```python
from build123d import *

# Parameters (mm, degrees)
SKETCH1_W           = 19.05
SKETCH1_H           = 38.1
SKETCH1_R           = 1.905
BOSS_EXTRUDE1_DEPTH = 3.81
BOSS_EXTRUDE2_DEPTH = 6.35
SKETCH3_W           = 10.16
SKETCH3_H           = 38.1
BOSS_EXTRUDE3_DEPTH = 2.54
CHAMFER1_SIZE       = 1.27


with BuildPart() as part:
    # Sketch1 → Boss-Extrude1 (new body)
    with BuildSketch(Plane(origin=(0, 0, 0), x_dir=(1, 0, 0), z_dir=(0, 1, 0))):
        with Locations((-4.445, -12.7)):
            Rectangle(SKETCH1_W, SKETCH1_H)
        with Locations(Location((0, 0, 0), (0, 0, 90))):
            Circle(SKETCH1_R, mode=Mode.SUBTRACT)
        with Locations(Location((0, -25.4, 0), (0, 0, 90))):
            Circle(SKETCH1_R, mode=Mode.SUBTRACT)
    extrude(amount=BOSS_EXTRUDE1_DEPTH)

    # Sketch2 → Boss-Extrude2 (add)
    with BuildSketch(Plane(origin=(0, 3.81, 0), x_dir=(1, 0, 0), z_dir=(0, 1, 0))):
        Polygon((-13.97, 6.35), (-13.97, -31.75), (-3.81, -31.75), (-3.81, 6.35), (-6.35, 6.35), (-6.35, -29.21), (-11.43, -29.21), (-11.43, 6.35), align=None)
    extrude(amount=BOSS_EXTRUDE2_DEPTH)

    # Sketch3 → Boss-Extrude3 (add)
    with BuildSketch(Plane(origin=(0, 10.16, 0), x_dir=(1, 0, 0), z_dir=(0, 1, 0))):
        with Locations((-8.89, -12.7)):
            Rectangle(SKETCH3_W, SKETCH3_H)
    extrude(amount=BOSS_EXTRUDE3_DEPTH)

    # Chamfer1
    chamfer1_edges = [part.edges().sort_by_distance(p)[0] for p in [
        (-6.35, 10.16, 11.43),
        (-11.43, 10.16, 11.43),
    ]]
    chamfer(chamfer1_edges, length=CHAMFER1_SIZE)


with BuildPart() as body_2:
    # Mirror1: mirrored copy
    add(part.part.mirror(Plane(origin=(5.08, 3.81, -6.35), x_dir=(0, 0, 1), z_dir=(-1, 0, 0))))


solid = body_2.part
```
Build history of the part. All positions in model axes, mm. A direction names the side the tool comes from. Coordinates: 2 decimals unless noted, no trailing zeros. Order: outer loops, then holes, each group sorted by start corner. A loop starts at its lowest first (then second) coordinate and runs counter-clockwise, first axis right, second up. Notation, with made-up numbers: (36, 76) -> (87, 76) arc R22 cw to (87, 87) -> close; hole circle Ø2 at (77, 30). An arc over 180 degrees is marked (long way). Answer in a Markdown table with one row per item. Add a question column.
Q1. Drop flat-ended pins along their axis: pin 1 (4.5 mm diameter, centred on x = 11, z = 5.5, fed in from +Y); pin 2 (2.5 mm diameter, centred on y = 9.5, z = 16, fed in from -X); pin 3 (3 mm diameter, centred on x = 12.5, z = 27.5, fed in from -Y). Give the stop position or say it passes through.
Q2. Which spindle directions (+Z, -Z, +X, -X, +Y, -Y) get a long thin tool onto all of the face, cutting with end or side? Do faces 1 (the face through (16.51, 6, 11)), 2 (the face through (10, 3.81, 12)), 3 (the face through (24.13, 6, 13)). Say none if no direction does.
Q3. Mould opens along X. For faces 4 (the face through (10.244, 1.878, 27.303)), 5 (the face through (17, 5, 31.75)), 6 (the face through (13.97, 8, 13)) say: +X half, -X half, draft (parallel to the pull), parting line (faces both ways), or undercut.
Q4. Band-saw the part on B-B, the plane z = 5.5. List the corners of the cut face in (x, y), then the cut area to 3 significant figures.
Q5. Band-saw the part on A-A, the plane z = 25.4. List the corners of the cut face in (x, y) (3 decimals).
Q6. Band-saw the part on C-C, the plane y = 2.5. List the corners of the cut face in (x, z) (3 decimals), then the cut area to 3 significant figures.
Q7. Band-saw the part on D-D, the plane x = 10.16. List the corners of the cut face in (y, z) (3 decimals).
Q8. Wall check: line 1 along X through (y, z) = (1.05, 0) (3 decimals); line 2 along X through (y, z) = (6.75, 9.5); line 3 along Y through (x, z) = (9.5, 9). Give the ranges that are in metal, low to high. Write a range as [from, to].
Answers follow:
| question | item | result |
|---|---|---|
| 1 | pin 1 | y = 3.81 |
| 1 | pin 2 | x = 13.97 |
| 1 | pin 3 | y = 0 |
| 2 | face 1 | -Z |
| 2 | face 2 | +Z, -Z, -X, +Y |
| 2 | face 3 | +Z, -Z, +X, +Y, -Y |
| 3 | face 4 | undercut |
| 3 | face 5 | draft |
| 3 | face 6 | -X half |
| 4 | outline | (5.08, 0) -> (24.13, 0) -> (24.13, 12.7) -> (13.97, 12.7) -> (13.97, 3.81) -> (5.08, 3.81) -> close; hole (16.51, 3.81) -> (21.59, 3.81) -> (21.59, 8.89) -> (20.32, 10.16) -> (17.78, 10.16) -> (16.51, 8.89) -> close |
| 4 | area | 132 mm^2 |
| 5 | outline | (5.08, 0) -> (8.255, 0) -> (8.255, 3.81) -> (5.08, 3.81) -> close; (12.065, 0) -> (24.13, 0) -> (24.13, 12.7) -> (13.97, 12.7) -> (13.97, 3.81) -> (12.065, 3.81) -> close; hole (16.51, 3.81) -> (21.59, 3.81) -> (21.59, 8.89) -> (20.32, 10.16) -> (17.78, 10.16) -> (16.51, 8.89) -> close |
| 6 | outline | (5.08, -6.35) -> (24.13, -6.35) -> (24.13, 31.75) -> (5.08, 31.75) -> close; hole circle Ø3.81 at (10.16, 0); hole circle Ø3.81 at (10.16, 25.4) |
| 6 | area | 703 mm^2 |
| 7 | outline | (0, -6.35) -> (3.81, -6.35) -> (3.81, -1.905) -> (0, -1.905) -> close; (0, 1.905) -> (3.81, 1.905) -> (3.81, 23.495) -> (0, 23.495) -> close; (0, 27.305) -> (3.81, 27.305) -> (3.81, 31.75) -> (0, 31.75) -> close |
| 8 | line 1 | [5.08, 8.255], [12.065, 24.13] |
| 8 | line 2 | [13.97, 16.51], [21.59, 24.13] |
| 8 | line 3 | [0, 3.81] |
